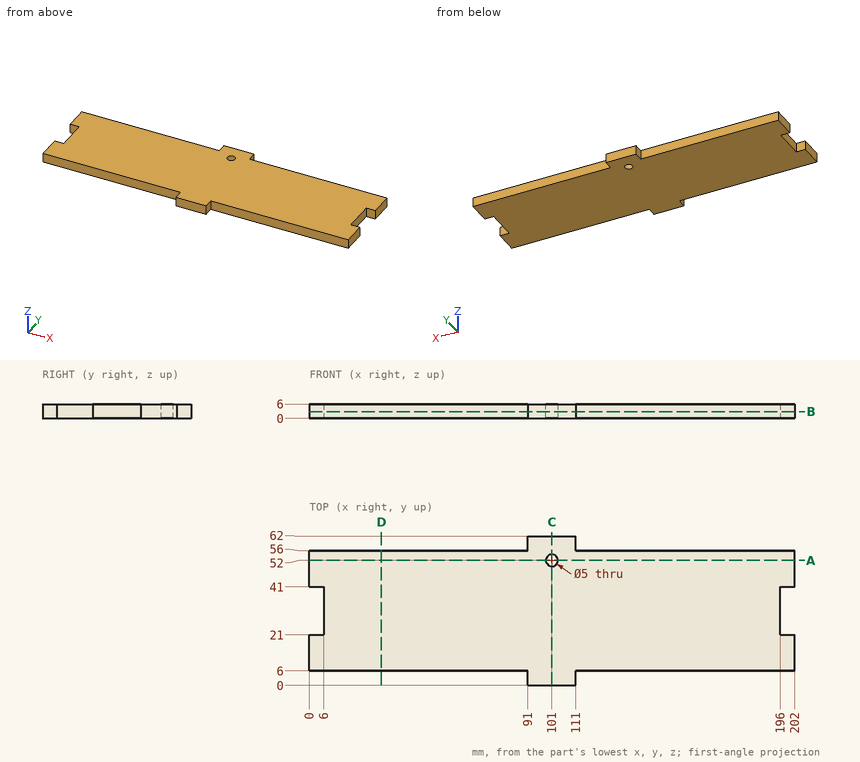
Check sheet for the drawn part. Datum: minimum x, y, z corner. Units: mm. Round coordinates to 2 decimals unless told otherwise and drop trailing zeros. Order: outer loops, then holes, each group sorted by start corner. A loop starts at its lowest first (then second) coordinate and runs counter-clockwise, first axis right, second up.
1) Go/stop test with flat-tipped pins: pin 1 Ø3 at (y, z) = (59, 4.5) entering from -X; pin 2 Ø1.8 at (x, z) = (4, 4) entering from +Y; pin 3 Ø1.8 at (y, z) = (60, 3) entering from +X. Record where each tip stops, or that it passes through.
2) Section check C-C (x = 101). Record the boundary of the cut face in (y, z), and give its area (3 significant figures).
3) Scan lines: line 1 (Y direction, x = 101, z = 2.5); line 2 (X direction, y = 52, z = 4.45); line 3 (Y direction, x = 53, z = 5.7). Record each from-to range of solid material in increasing order.
4) Section check A-A (y = 52). Record the boundary of the cut face in (x, z), and give its area (3 significant figures).
5) Section check D-D (x = 30). Record the boundary of the cut face in (y, z).
6) Section check B-B (z = 2.85). Record the boundary of the cut face in (x, y).
Result:
1. pin 1: stops at x = 91
1. pin 2: stops at y = 56
1. pin 3: stops at x = 111
2. outline: (0, 0) - (49.5, 0) - (49.5, 6) - (0, 6) - close; (54.5, 0) - (62, 0) - (62, 6) - (54.5, 6) - close
2. area: 342 mm2
3. line 1: y = 0 to 49.5, 54.5 to 62
3. line 2: x = 0 to 98.5, 103.5 to 202
3. line 3: y = 6 to 56
4. outline: (0, 0) - (98.5, 0) - (98.5, 6) - (0, 6) - close; (103.5, 0) - (202, 0) - (202, 6) - (103.5, 6) - close
4. area: 1,180 mm2
5. outline: (6, 0) - (56, 0) - (56, 6) - (6, 6) - close
6. outline: (0, 6) - (91, 6) - (91, 0) - (111, 0) - (111, 6) - (202, 6) - (202, 21) - (196, 21) - (196, 41) - (202, 41) - (202, 56) - (111, 56) - (111, 62) - (91, 62) - (91, 56) - (0, 56) - (0, 41) - (6, 41) - (6, 21) - (0, 21) - close; hole circle Ø5 at (101, 52)
